Can you work these out from the model? Positions are in its coordinate system, mm. Face numbers are marked on the shaded views. A direction names the side the tool comes from. Give positions to 0.01 mm unless a question says otherwise; leave off trailing zeros. Loops run counter-clockwise (first coordinate to the right, second up) from the corner with the lowest first, then second, coordinate; pieces in that order, holes last. Notation, with made-up numbers: M 18,-4 L 50,-4 A12 ccw 50,11 Z; hole C -15.75,37.5 d1. An arc over 180 degrees is marked long. Put each result on its own line as item: value. Start each with the question number.
1) Imagine slicing it at A-A (y = 14). Write out the boundary of the cut face in (x, z).
2) For the marked faces 4, 5 and 6, which set-ups out of +Z, -Z, +X, -X, +Y, -Y let a thin tool reach every point of the face, with its end or its side?
3) Imagine slicing it at C-C (x = 4). Write out the boundary of the cut face in (y, z).
4) Imagine slicing it at B-B (z = 2.25). Write out the boundary of the cut face in (x, y), then the cut area to 3 significant figures.
5) Please list where these lines run through material, in increasing order: line 1 along X through (y, z) = (9.5, 13); line 2 along Y through (x, z) = (6.25, 1.25); line 3 along X through (y, z) = (12, 18.6). Write a range as from..to.
6) For P1, Ø2, axis at x = 3.5, y = 12.5, coming from the -Z side; P2, Ø2.5, axis at x = 4, z = 12.5, coming from the -Y side, each with a flat end and sliding along its axis, tell me the tip position at first contact or that it passes through.
7) Imagine slicing it at D-D (y = 12). Write out the boundary of the cut face in (x, z), then the cut area to 4 significant figures.
8) If we mould it in two halves opening along Y, with no side actions, what happens to the marked faces 1, 2 and 3? For each: +Y half, -Y half, draft (parallel to the pull), parting line (faces both ways), or undercut.
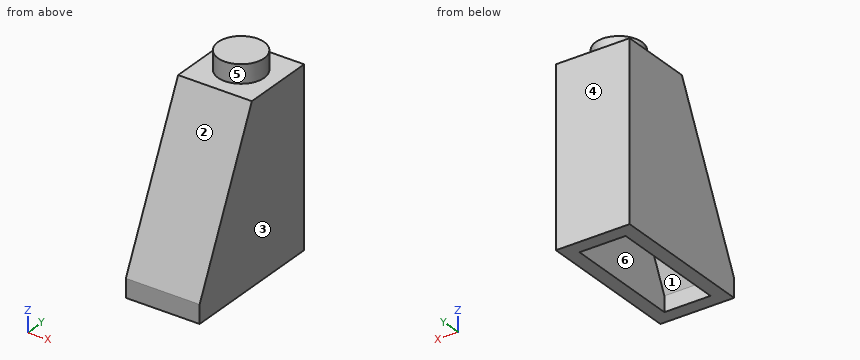
from build123d import *

# Parameters (mm, degrees)
F1_DEPTH = 4
F3_DEPTH = 2.5
F5_R     = 2.5
F6_DEPTH = 2
F7_R     = 1.25
F8_DEPTH = 20


with BuildPart() as f1:
    # F0 (on Right) → F1 (new body)
    with BuildSketch(Plane.YZ):
        Polygon((0, 2), (0, 0), (16, 0), (16, 19), (8, 19), align=None)
    extrude(amount=F1_DEPTH)

    # F2 (on face) → F3 (cut)
    with BuildSketch(Plane.YZ.offset(4)):
        Polygon((14.5, 0), (14.5, 17.5), (8.951908, 17.5), (1.5, 1.664695), (1.5, 0), align=None)
    extrude(amount=-F3_DEPTH, mode=Mode.SUBTRACT)

    # F4: F1 across face


with BuildPart() as f1_1:
    add(f1.part)
    add(f1.part.mirror(Plane(origin=(4, 9.86239, 10.544939), x_dir=(0, 1, 0), z_dir=(1, 0, 0))))

    # F5 (on face) → F6 (join)
    with BuildSketch(Plane.XY.offset(19)):
        with Locations((4, 12)):
            Circle(F5_R)
    extrude(amount=F6_DEPTH)

    # F7 (on face) → F8 (cut)
    with BuildSketch(Plane(origin=(0, 0, 0), x_dir=(1, 0, 0), z_dir=(0, 0, -1))):
        with Locations((4, -12)):
            Circle(F7_R)
    extrude(amount=-F8_DEPTH, mode=Mode.SUBTRACT)


solid = f1_1.part
Recorded:
1. outline: M 0,0 L 1.5,0 L 1.5,17.5 L 6.5,17.5 L 6.5,0 L 8,0 L 8,19 L 5.5,19 L 5.5,21 L 2.5,21 L 2.5,19 L 0,19 Z
2. face 4: +Z, -Z, +X, -X, +Y
2. face 5: +Z
2. face 6: -Z
3. outline: M 0,0 L 1.5,0 L 1.5,1.66 L 8.95,17.5 L 10.75,17.5 L 10.75,20 L 13.25,20 L 13.25,17.5 L 14.5,17.5 L 14.5,0 L 16,0 L 16,19 L 14.5,19 L 14.5,21 L 9.5,21 L 9.5,19 L 8,19 L 0,2 Z
4. outline: M 0,0.12 L 8,0.12 L 8,16 L 0,16 Z; hole M 1.5,1.78 L 6.5,1.78 L 6.5,14.5 L 1.5,14.5 Z
4. area: 63.4 mm²
5. line 1: 0..1.5, 6.5..8
5. line 2: 0..1.5, 14.5..16
5. line 3: 0..2.75, 5.25..8
6. P1: z = 17.5
6. P2: y = 4.35
7. outline: M 0,0 L 1.5,0 L 1.5,17.5 L 2.75,17.5 L 2.75,20 L 5.25,20 L 5.25,17.5 L 6.5,17.5 L 6.5,0 L 8,0 L 8,19 L 6.5,19 L 6.5,21 L 1.5,21 L 1.5,19 L 0,19 Z
7. area: 68.25 mm²
8. face 1: undercut
8. face 2: -Y half
8. face 3: draft
